The model under review builds one solid part; all positions refer to its coordinate system, in mm. Give positions to 0.01 mm unless a question says otherwise; leave off trailing zeros. Order: outer loops, then holes, each group sorted by start corner. A loop starts at its lowest first (then second) coordinate and runs counter-clockwise, first axis right, second up. Notation, with made-up numbers: (-29, 83) - (17, 83) arc R28 ccw to (17, 105) - close; hole circle Ø8 at (42, 62.25). An arc over 180 degrees is marked (long way). Write item = value, one per line. Start each with the question number.
1. For P1, Ø4.5, axis at x = -127, z = 12.7, coming from the +Y side; P2, Ø6.5, axis at x = 127, z = 12.7, coming from the +Y side; P3, Ø5, axis at x = -106.5, z = 21.5, coming from the +Y side, all flat-tipped, find the tip position at first contact; note any pin that passes through.
2. We need section A-A, the plane x = 127. Give the boundary of the cut face in (y, z).
3. We need section C-C, the plane z = 12.7. Give the boundary of the cut face in (x, y), and give its area (3 significant figures).
4. We need section D-D, the plane x = 87. Give the boundary of the cut face in (y, z).
5. Wall thickness on probe 1 along Z at (x, y) = (-127, 5); probe 2 along Y at (x, z) = (-1.5, 15.75); probe 3 along Y at (x, z) = (-63, 2.25): over which ranges is each line inside the solid? List them lowest first.
from build123d import *

# Parameters (mm, degrees)
BOSS_EXTRUDE3_DEPTH = 25.4
SKETCH2_R           = 4.7625
CUT_EXTRUDE1_DEPTH  = 25.4
SKETCH3_R           = 2.5527
CUT_EXTRUDE2_DEPTH  = 12.7


with BuildPart() as part:
    # Sketch1 → Boss-Extrude3 (new body)
    with BuildSketch(Plane.XY):
        with BuildLine():
            ThreePointArc((-158.75, 0), (0, 19.015868295), (158.75, 0))
            Line((158.75, 0), (-158.75, 0))
        make_face()
    extrude(amount=BOSS_EXTRUDE3_DEPTH)

    # Sketch2 → Cut-Extrude1 (cut)
    with BuildSketch(Plane.XZ):
        with Locations((-180.975, 12.7)):
            Circle(SKETCH2_R)
        with Locations((180.975, 12.7)):
            Circle(SKETCH2_R)
    extrude(amount=-CUT_EXTRUDE1_DEPTH, mode=Mode.SUBTRACT)

    # Sketch3 → Cut-Extrude2 (cut)
    with BuildSketch(Plane.XZ):
        with Locations(Location((-127, 12.7, 0), (0, 0, 270))):
            Circle(SKETCH3_R)
        with Locations(Location((127, 12.7, 0), (0, 0, 270))):
            Circle(SKETCH3_R)
    extrude(amount=-CUT_EXTRUDE2_DEPTH, mode=Mode.SUBTRACT)


solid = part.part
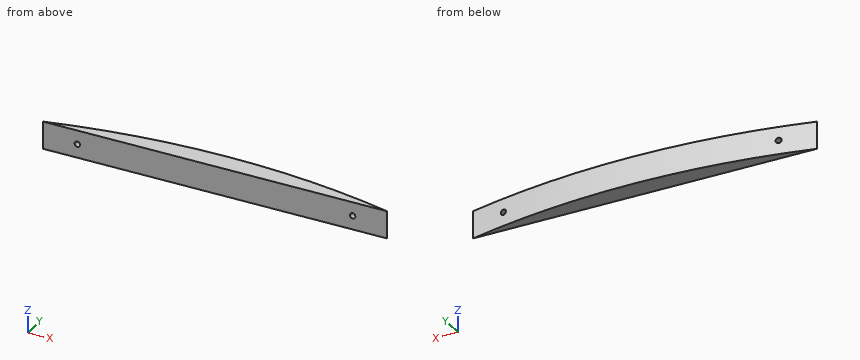
Model answer:
q1.P1 = through
q1.P2 = 7.53
q1.P3 = 10.92
q2.outline = (0, 0) - (6.91, 0) - (6.91, 10.15) - (0, 10.15) - close; (0, 15.25) - (6.91, 15.25) - (6.91, 25.4) - (0, 25.4) - close
q3.outline = (-158.75, 0) - (-129.55, 0) - (-129.55, 6.41) arc R672.15 ccw to start; (-124.45, 0) - (124.45, 0) - (124.45, 7.39) arc R672.15 ccw to (-124.45, 7.39) - close; (129.55, 0) - (158.75, 0) arc R672.15 ccw to (129.55, 6.41) - close
q3.area = 3,970 mm2
q4.outline = (0, 0) - (13.36, 0) - (13.36, 25.4) - (0, 25.4) - close
q5.probe_1 = 0 to 10.15, 15.25 to 25.4
q5.probe_2 = 0 to 19.01
q5.probe_3 = 0 to 16.06
